Check sheet for the modelled part. Datum: model origin and axes. Units: mm. A direction names the side the tool comes from. Give positions to 0.01 mm unless a question says otherwise; leave off trailing zeros. Order: outer loops, then holes, each group sorted by start corner. A loop starts at its lowest first (then second) coordinate and runs counter-clockwise, first axis right, second up. Notation, with made-up numbers: (65.5, -20) -> (70.5, -20) arc R10 ccw to (70.5, -7) -> close; hole circle Ø9 at (38.5, -28.75). An arc over 180 degrees is marked (long way). Answer in a Markdown table with one row per item. Add a question column.
(1) Cross-section at B-B (x = 54.5). Record the cut outline in (y, z), then the cut area to 4 significant figures.
(2) Cross-section at D-D (z = 1.55). State how many separate pieces and enclosed holes the cut face has, then the cut area to 3 significant figures.
(3) Thickness scan on L1, parallel to Y at x = -63.5, z = 1.2; L2, parallel to Y at x = -102.5, z = 2.3; L3, parallel to X at y = 52.5, z = 1.6. Record the ranges inside material, lowest first. Write a range as [from, to].
(4) Go/stop test with flat-tipped pins: pin 1 (2.5 mm diameter, centred on x = 13.79, y = 5, fed in from +Z); pin 2 (1 mm diameter, centred on y = -60.5, z = 0.5, fed in from -X); pin 3 (1 mm diameter, centred on x = -22, z = 2.5, fed in from +Y); pin 4 (1.5 mm diameter, centred on x = 182.5, z = 1, fed in from +Y). Record where each tip stops, or that it passes through.
(5) Cross-section at C-C (y = -15). Record the cut outline in (x, z).
(6) Release check for a two-part mould opening along X. For faces 3 (the face through (-14.095, -53.394, 1.521)), 4 (the face through (143.751, 57.348, 1.479)), 5 (the face through (76, -9, 0)) record: released by +X, released by -X, zero draft, split by the parting line, or undercut.
(7) Cross-section at A-A (y = 24). Record the cut outline in (x, z).
(8) Set-up check for faces 1 (the face through (154.51, 19.69, 1.52)), 2 (the face through (-4.65, 73.926, 1.521)): record each of +Z, -Z, +X, -X, +Y, -Y from which the full face is reachable in a straight line by a thin tool's end or side.
```python
from build123d import *

# Parameters (mm, degrees)
SKETCH1_W           = 184.414327478
SKETCH1_H           = 83.61431582
BOSS_EXTRUDE1_DEPTH = 3
SKETCH2_R           = 3
CUT_EXTRUDE1_DEPTH  = 70
SKETCH3_R           = 11.25
CUT_EXTRUDE2_DEPTH  = 3
SKETCH4_R           = 1.6
BOSS_EXTRUDE2_DEPTH = 3
CUT_EXTRUDE3_DEPTH  = 10
SKETCH6_R           = 1.6
CUT_EXTRUDE4_DEPTH  = 3
FILLET1_R           = 1.5
SKETCH8_R           = 1.6
CUT_EXTRUDE6_DEPTH  = 12
SKETCH9_R           = 2.15
CUT_EXTRUDE7_DEPTH  = 12
BOSS_EXTRUDE3_DEPTH = 3
SKETCH12_R          = 1.6
CUT_EXTRUDE8_DEPTH  = 10
SKETCH13_R          = 1
CUT_EXTRUDE9_DEPTH  = 10


with BuildPart() as part:
    # Sketch1 → Boss-Extrude1 (new body)
    with BuildSketch(Plane.XY):
        with Locations((112.494062572, 5.79284209)):
            Rectangle(SKETCH1_W, SKETCH1_H)
    extrude(amount=BOSS_EXTRUDE1_DEPTH)

    # Sketch2 → Cut-Extrude1 (cut)
    with BuildSketch(Plane(origin=(0, 0, 0), x_dir=(-1, 0, 0), z_dir=(0, 0, -1))):
        with Locations((-24.116880081, 24)):
            Circle(SKETCH2_R)
    extrude(amount=-CUT_EXTRUDE1_DEPTH, mode=Mode.SUBTRACT)

    # Sketch3 → Cut-Extrude2 (cut)
    with BuildSketch(Plane.XY.offset(3)):
        with Locations((144.116880081, 24)):
            Circle(SKETCH3_R)
    extrude(amount=-CUT_EXTRUDE2_DEPTH, mode=Mode.SUBTRACT)

    # Sketch4 → Boss-Extrude2 (add)
    with BuildSketch(Plane.XY.offset(3)):
        with BuildLine():
            Line((-61.543119919, 56), (-61.543119919, 34))
            Line((-61.543119919, 34), (-72.043119919, 34))
            ThreePointArc((-72.043119919, 34), (-73.457333481, 33.414213562), (-74.043119919, 32))
            Line((-74.043119919, 32), (-74.043119919, 6))
            ThreePointArc((-74.043119919, 6), (-73.457333481, 4.585786438), (-72.043119919, 4))
            Line((-72.043119919, 4), (-61.543119919, 4))
            Line((-61.543119919, 4), (-61.543119919, -26))
            Line((-61.543119919, -26), (34.701226311, -81.566699204))
            Line((34.701226311, -81.566699204), (204.701226311, -81.566699204))
            Line((204.701226311, -81.566699204), (204.701226311, -36.01431582))
            Line((204.701226311, -36.01431582), (20.286898833, -36.01431582))
            Line((20.286898833, -36.01431582), (20.286898833, 47.6))
            Line((20.286898833, 47.6), (40.948393205, 47.6))
            Line((40.948393205, 47.6), (-51.543119919, 101))
            Line((-51.543119919, 101), (-121.543119919, 101))
            Line((-121.543119919, 101), (-121.543119919, 56))
            Line((-121.543119919, 56), (-61.543119919, 56))
        make_face()
        with Locations((-71.043119919, 31)):
            Circle(SKETCH4_R, mode=Mode.SUBTRACT)
        with Locations((-71.043119919, 7)):
            Circle(SKETCH4_R, mode=Mode.SUBTRACT)
    extrude(amount=-BOSS_EXTRUDE2_DEPTH)

    # Sketch5 → Cut-Extrude3 (cut)
    with BuildSketch(Plane.XY.offset(3)):
        with BuildLine():
            Line((8.286898833, 8.5), (-51.373138671, 8.5))
            ThreePointArc((-51.373138671, 8.5), (-52.433798843, 8.939339828), (-52.873138671, 10))
            Line((-52.873138671, 10), (-52.873138671, 38))
            ThreePointArc((-52.873138671, 38), (-52.433798843, 39.060660172), (-51.373138671, 39.5))
            Line((-51.373138671, 39.5), (-42.743119919, 39.5))
            Line((-42.743119919, 39.5), (-42.743119919, 62.05))
            ThreePointArc((-42.743119919, 62.05), (-43.273450005, 63.330330086), (-41.993119919, 62.8))
            Line((-41.993119919, 62.8), (-1.093119919, 62.8))
            ThreePointArc((-1.093119919, 62.8), (0.187210167, 63.330330086), (-0.343119919, 62.05))
            Line((-0.343119919, 62.05), (-0.343119919, 39.5))
            Line((-0.343119919, 39.5), (8.286898833, 39.5))
            ThreePointArc((8.286898833, 39.5), (9.347559005, 39.060660172), (9.786898833, 38))
            Line((9.786898833, 38), (9.786898833, 10))
            ThreePointArc((9.786898833, 10), (9.347559005, 8.939339828), (8.286898833, 8.5))
        make_face()
    extrude(amount=-CUT_EXTRUDE3_DEPTH, mode=Mode.SUBTRACT)

    # Sketch6 → Cut-Extrude4 (cut)
    with BuildSketch(Plane.XY.offset(3)):
        with Locations((13.786898833, 5)):
            Circle(SKETCH6_R)
        with Locations((13.786898833, 39.6)):
            Circle(SKETCH6_R)
        with Locations((-56.873138671, 5)):
            Circle(SKETCH6_R)
        with Locations((-56.873138671, 39.6)):
            Circle(SKETCH6_R)
    extrude(amount=-CUT_EXTRUDE4_DEPTH, mode=Mode.SUBTRACT)

    # Fillet1
    fillet1_edges = [part.edges().sort_by_distance(p)[0] for p in [
        (-61.543119919, 4, 1.5),
        (-61.543119919, 34, 1.5),
    ]]
    fillet(fillet1_edges, radius=FILLET1_R)

    # Sketch8 → Cut-Extrude6 (cut)
    with BuildSketch(Plane.XY.offset(3)):
        with Locations((-90.243119919, 94)):
            Circle(SKETCH8_R)
        with Locations((-90.243119919, 64)):
            Circle(SKETCH8_R)
    extrude(amount=-CUT_EXTRUDE6_DEPTH, mode=Mode.SUBTRACT)

    # Sketch9 → Cut-Extrude7 (cut)
    with BuildSketch(Plane(origin=(0, 0, 0), x_dir=(-1, 0, 0), z_dir=(0, 0, -1))):
        with Locations((-172.128729044, 31.505752308)):
            Circle(SKETCH9_R)
        with Locations((-123.610783427, 44.506096654)):
            Circle(SKETCH9_R)
        with Locations((-136.611127773, -4.011848962)):
            Circle(SKETCH9_R)
    extrude(amount=-CUT_EXTRUDE7_DEPTH, mode=Mode.SUBTRACT)

    # Sketch10 → Boss-Extrude3 (add)
    with BuildSketch(Plane(origin=(0, 0, 0), x_dir=(-1, 0, 0), z_dir=(0, 0, -1))):
        with BuildLine():
            Line((-167.680888654, 47.6), (-120.552871509, 47.6))
            ThreePointArc((-120.552871509, 47.6), (-144.116880081, 57.35), (-167.680888654, 47.6))
        make_face()
    extrude(amount=-BOSS_EXTRUDE3_DEPTH)

    # Sketch12 → Cut-Extrude8 (cut)
    with BuildSketch(Plane.XY.offset(3)):
        with Locations((23.701226311, -61.566699204)):
            Circle(SKETCH12_R)
        with BuildLine():
            ThreePointArc((110.101226311, -61.566699204), (109.784541603, -68.957425033), (108.836808989, -76.293971931))
            ThreePointArc((108.836808989, -76.293971931), (110.140666581, -78.143284068), (111.989978718, -76.839426476))
            ThreePointArc((111.989978718, -76.839426476), (112.97281254, -69.231155619), (113.301226311, -61.566699204))
            ThreePointArc((113.301226311, -61.566699204), (111.701226311, -59.966699204), (110.101226311, -61.566699204))
        make_face()
    extrude(amount=-CUT_EXTRUDE8_DEPTH, mode=Mode.SUBTRACT)

    # Sketch13 → Cut-Extrude9 (cut)
    with BuildSketch(Plane(origin=(0, 0, 0), x_dir=(-1, 0, 0), z_dir=(0, 0, -1))):
        with Locations((-163.256880081, -19.666699204)):
            Circle(SKETCH13_R)
        with Locations((-163.256880081, -37.666699204)):
            Circle(SKETCH13_R)
        with Locations((-118.056880081, -19.666699204)):
            Circle(SKETCH13_R)
        with Locations((-118.056880081, -37.666699204)):
            Circle(SKETCH13_R)
    extrude(amount=-CUT_EXTRUDE9_DEPTH, mode=Mode.SUBTRACT)


solid = part.part
```
Answer below:
| question | item | result |
|---|---|---|
| 1 | outline | (-81.57, 0) -> (47.6, 0) -> (47.6, 3) -> (-81.57, 3) -> close |
| 1 | area | 387.5 mm² |
| 2 | separate pieces | 1 |
| 2 | enclosed holes | 20 |
| 2 | area | 34,600 mm² |
| 3 | L1 | y = [4, 34], [56, 101] |
| 3 | L2 | y = [56, 101] |
| 3 | L3 | x = [-61.54, -42.74], [-0.34, 32.46], [126.8, 161.44] |
| 4 | pin 1 | passes through |
| 4 | pin 2 | stops at x = -2.65 |
| 4 | pin 3 | stops at y = 84.23 |
| 4 | pin 4 | stops at y = 47.6 |
| 5 | outline | (-61.54, 0) -> (204.7, 0) -> (204.7, 3) -> (-61.54, 3) -> close |
| 6 | face 3 | released by -X |
| 6 | face 4 | undercut |
| 6 | face 5 | zero draft |
| 7 | outline | (-74.04, 0) -> (-52.87, 0) -> (-52.87, 3) -> (-74.04, 3) -> close; (9.79, 0) -> (21.12, 0) -> (21.12, 3) -> (9.79, 3) -> close; (27.12, 0) -> (132.87, 0) -> (132.87, 3) -> (27.12, 3) -> close; (155.37, 0) -> (204.7, 0) -> (204.7, 3) -> (155.37, 3) -> close |
| 8 | face 1 | +Z, -Z |
| 8 | face 2 | +Z, -Z, +Y |
